from build123d import *

# Parameters (mm, degrees)
CYLINDER372_R     = 2
CYLINDER372_DEPTH = 70
CYLINDER373_R     = 2
CYLINDER373_DEPTH = 70
CYLINDER369_R     = 4
CYLINDER369_DEPTH = 5
BOX463_W          = 2.7
BOX463_H          = 20.1
BOX463_DEPTH      = 5
BOX459_W          = 20
BOX459_H          = 52
BOX459_DEPTH      = 3
FILLET016_R       = 8


with BuildPart() as cylinder372:
    # Cylinder372 → Cylinder372 (new body)
    with BuildSketch(Plane(origin=(-90, -103, -10), x_dir=(1, 0, 0), z_dir=(0, 0, 1))):
        Circle(CYLINDER372_R)
    extrude(amount=CYLINDER372_DEPTH)


with BuildPart() as fusion369:
    # Cylinder373 → Cylinder373 (new body)
    with BuildSketch(Plane(origin=(-90, -61, -10), x_dir=(1, 0, 0), z_dir=(0, 0, 1))):
        Circle(CYLINDER373_R)
    extrude(amount=CYLINDER373_DEPTH)

    # Fusion369: union Cylinder372
    add(cylinder372.part)


with BuildPart() as fusion369_1:
    # Fusion369 placement: moved
    add(fusion369.part.moved(Location((114, 0, 0))))


with BuildPart() as cylinder369:
    # Cylinder369 → Cylinder369 (new body)
    with BuildSketch(Plane(origin=(24, -70, 39), x_dir=(1, 0, 0), z_dir=(0, 0, 1))):
        Circle(CYLINDER369_R)
    extrude(amount=CYLINDER369_DEPTH)


with BuildPart() as box463:
    # Box463 → Box463 (new body)
    with BuildSketch(Plane(origin=(22.5, -98.1, 39), x_dir=(1, 0, 0), z_dir=(0, 0, 1))):
        with Locations((1.35, 10.05)):
            Rectangle(BOX463_W, BOX463_H)
    extrude(amount=BOX463_DEPTH)


with BuildPart() as cut402:
    # Box459 → Box459 (new body)
    with BuildSketch(Plane(origin=(14, -108, 40.1), x_dir=(1, 0, 0), z_dir=(0, 0, 1))):
        with Locations((10, 26)):
            Rectangle(BOX459_W, BOX459_H)
    extrude(amount=BOX459_DEPTH)

    # Cut397: cut Box463
    add(box463.part, mode=Mode.SUBTRACT)

    # Fillet016
    fillet016_edges = [cut402.edges().sort_by_distance(p)[0] for p in [
        (14, -108, 41.6),
        (14, -56, 41.6),
        (34, -108, 41.6),
        (34, -56, 41.6),
    ]]
    fillet(fillet016_edges, radius=FILLET016_R)

    # Cut400: cut Cylinder369
    add(cylinder369.part, mode=Mode.SUBTRACT)

    # Cut402: cut Fusion369
    add(fusion369_1.part, mode=Mode.SUBTRACT)


solid = cut402.part
Verification items for the finished model (mm, model axes). A direction names the side the tool comes from. Coordinates: 2 decimals unless noted, no trailing zeros. Order: outer loops, then holes, each group sorted by start corner. A loop starts at its lowest first (then second) coordinate and runs counter-clockwise, first axis right, second up.
Item 1: Section check A-A, the plane y = -70. Enter the section's corners in (x, z), then the cut area to 3 significant figures.
Filled in:
outline: (14, 40.1) - (20, 40.1) - (20, 43.1) - (14, 43.1) - close; (28, 40.1) - (34, 40.1) - (34, 43.1) - (28, 43.1) - close
area: 36.0 mm2
Item 2: Material ranges on L1, parallel to Y at x = 24, z = 42.1; L2, parallel to X at y = -79, z = 42.75; L3, parallel to X at y = -103, z = 41.3, recorded low to high.
Filled in:
L1: y = -108 to -105, -101 to -98.1, -78 to -74, -66 to -63, -59 to -56
L2: x = 14 to 22.5, 25.2 to 34
L3: x = 14.58 to 22, 26 to 33.42
Item 3: Depth check by flat-ended pin: pin 1 (1 mm diameter, centred on x = 20.5, z = 42, fed in from +Y). Enter the tip coordinate at first touch or a pass-through.
Filled in:
pin 1: stops at y = -56.06
Item 4: Access from +Z, -Z, +X, -X, +Y, -Y to the whole of each face (thin tool, end or side, straight path). Record for faces 5 (the face through (16.281, -58.406, 41.621)), 6 (the face through (22.5, -88, 42)).
Filled in:
face 5: +Z, -Z, -X, +Y
face 6: +Z, -Z
Item 5: Section check D-D, the plane x = 24. Enter the section's corners in (y, z), then the cut area to 3 significant figures.
Filled in:
outline: (-108, 40.1) - (-105, 40.1) - (-105, 43.1) - (-108, 43.1) - close; (-101, 40.1) - (-98.1, 40.1) - (-98.1, 43.1) - (-101, 43.1) - close; (-78, 40.1) - (-74, 40.1) - (-74, 43.1) - (-78, 43.1) - close; (-66, 40.1) - (-63, 40.1) - (-63, 43.1) - (-66, 43.1) - close; (-59, 40.1) - (-56, 40.1) - (-56, 43.1) - (-59, 43.1) - close
area: 47.7 mm2
Item 6: Section check C-C, the plane x = 21.5. Enter the section's corners in (y, z), then the cut area to 3 significant figures.
Filled in:
outline: (-107.98, 40.1) - (-73.12, 40.1) - (-73.12, 43.1) - (-107.98, 43.1) - close; (-66.88, 40.1) - (-56.02, 40.1) - (-56.02, 43.1) - (-66.88, 43.1) - close
area: 137 mm2
Item 7: Release check for a two-part mould opening along Y. For faces 1 (the face through (34, -82, 42)), 2 (the face through (25.2, -88, 42)), 3 (the face through (24, -108, 42)), 4 (the face through (24, -56, 42)) record: +Y half, -Y half, draft (parallel to the pull), parting line (faces both ways), or undercut.
Filled in:
face 1: draft
face 2: undercut
face 3: -Y half
face 4: +Y half
Item 8: Section check B-B, the plane z = 40.95. Enter the section's corners in (x, y), then the cut area to 3 significant figures.
Filled in:
outline: (14, -100) arc R8 ccw to (22, -108) - (26, -108) arc R8 ccw to (34, -100) - (34, -64) arc R8 ccw to (26, -56) - (22, -56) arc R8 ccw to (14, -64) - close; hole circle Ø8 at (24, -70); hole circle Ø4 at (24, -103); hole circle Ø4 at (24, -61); hole (22.5, -98.1) - (25.2, -98.1) - (25.2, -78) - (22.5, -78) - close
area: 855 mm2
